Part model, mm, in its own coordinate system. A direction names the side the tool comes from. Coordinates: 2 decimals unless noted, no trailing zeros. Loops run counter-clockwise (first coordinate to the right, second up) from the corner with the lowest first, then second, coordinate; pieces in that order, holes last. Notation, with made-up numbers: (77.5, -31.5) - (112.5, -31.5) arc R29 ccw to (112.5, -3.5) - close; hole circle Ø2 at (26, 47). An arc over 180 degrees is marked (long way). Use a Markdown table: item, result. Add a question column.
1) Tool access for faces 4 (the face through (-2.5, -1.1, 8.7)), 5 (the face through (12, -7, 8)), 6 (the face through (13, 5, 8)), 7 (the face through (-1, -7, 8)), 8 (the face through (1.5, -1.1, 8.7)): list every direction of +Z, -Z, +X, -X, +Y, -Y with a clear straight run to the whole face (end or side of a thin tool).
2) Band-saw the part on C-C (x = 1). Give the cut face in (y, z), plus the area to 3 significant figures.
3) Drop flat-ended pins along their axis: P1, Ø2, axis at x = -0.5, z = 9, coming from the -Y side; P2, Ø1, axis at x = -17.5, y = -8.5, coming from the +Z side; P3, Ø2, axis at x = 11.5, z = 5.5, coming from the +Y side; P4, Ø1, axis at y = -9.5, z = 4, coming from the +X side. Give the stop position or say it passes through.
4) Band-saw the part on D-D (z = 16.25). Give the cut face in (x, y), plus the area to 3 significant figures.
5) Probe probe 1 along Y at (x, z) = (13.5, 11.85); probe 2 along X at (y, z) = (4, 9); probe 3 along Z at (x, y) = (3, 9). List the from-to ranges inside material, lowest first. Write a range as [from, to].
6) Pull direction X, two halves, no side cores. Call faces 1 (the face through (-5, -2, 0)), 2 (the face through (10.5, -0.9, 8.7)), 3 (the face through (-24.5, -9, 1)): +X half, -X half, draft (parallel to the pull), parting line (faces both ways), or undercut.
7) Band-saw the part on B-B (z = 5.25). Give the cut face in (x, y), plus the area to 4 significant figures.
8) Band-saw the part on A-A (z = 11.85). Give the cut face in (x, y).
from build123d import *

# Parameters (mm, degrees)
ESBO_O1_W                  = 10
ESBO_O1_H                  = 4
RESSALTO_EXTRUS_O1_DEPTH   = 3
ESBO_O1_8_W                = 4
ESBO_O1_8_H                = 12
RESSALTO_EXTRUS_O2_DEPTH   = 18
CORTE_EXTRUS_O1_DEPTH      = 47.968074263
CORTE_EXTRUS_O1_DEPTH_BACK = 47.968074263
ESBO_O2_R                  = 3
ESBO_O1_9_W                = 10
ESBO_O1_9_H                = 4
RESSALTO_EXTRUS_O3_DEPTH   = 8
CHANFRO1_SIZE              = 5


with BuildPart() as part:
    # Esboço1 → Ressalto-extrusão1 (new body)
    # profile 1 of 2: a face of its own
    with BuildSketch(Plane.XY):
        Polygon((-24.5, -15), (-24.5, -19), (-15.5, -19), (4.5, -19), (4.5, -15), (14.5, -15), (14.5, -7), (10.5, -7), (10.5, 5), (14.5, 5), (14.5, 15), (1.5, 15), (-1.605263158, 15), (-24.5, 0), align=None)
        with BuildLine():
            ThreePointArc((-15.5, -16.5), (-16.560660172, -16.060660172), (-17, -15))
            ThreePointArc((-17, -15), (-15.5, -13.5), (-14, -15))
            ThreePointArc((-14, -15), (-14.439339828, -16.060660172), (-15.5, -16.5))
        make_face(mode=Mode.SUBTRACT)
        Polygon((-2.5, 5), (1.5, 5), (1.5, -7), (-2.5, -7), (-2.5, 0), align=None, mode=Mode.SUBTRACT)
    # profile 2 of 2: a face of its own
    with BuildSketch(Plane.XY):
        with Locations((9.5, -17)):
            Rectangle(ESBO_O1_W, ESBO_O1_H)
    extrude(amount=RESSALTO_EXTRUS_O1_DEPTH)

    # Esboço1<8> → Ressalto-extrusão2 (add)
    with BuildSketch(Plane.XY):
        Polygon((10.5, -7), (14.5, -7), (14.5, -2), (14.5, 5), (10.5, 5), align=None)
        with Locations((-0.5, -1)):
            Rectangle(ESBO_O1_8_W, ESBO_O1_8_H)
    extrude(amount=RESSALTO_EXTRUS_O2_DEPTH)

    # Esboço2 → Corte-extrusão1 (cut, two sides: drawn at the far end of the back side and taken through both)
    with BuildSketch(Plane(origin=(14.5, 0, 0), x_dir=(0, 0, -1), z_dir=(1, 0, 0)).offset(-CORTE_EXTRUS_O1_DEPTH_BACK)):
        with BuildLine():
            ThreePointArc((-18, -1), (-16.652343178, 2.841874542), (-13.2, 5))
            Line((-13.2, 5), (-18, 5))
            Line((-18, 5), (-18, -1))
        make_face()
        with BuildLine():
            ThreePointArc((-13.2, -7), (-16.652343178, -4.841874542), (-18, -1))
            Line((-18, -1), (-18, -7))
            Line((-18, -7), (-13.2, -7))
        make_face()
        with Locations(Location((-11.85, -1, 0), (0, 0, 180))):
            Circle(ESBO_O2_R)
    extrude(amount=CORTE_EXTRUS_O1_DEPTH + CORTE_EXTRUS_O1_DEPTH_BACK, mode=Mode.SUBTRACT)

    # Esboço1<9> → Ressalto-extrusão3 (add)
    with BuildSketch(Plane.XY):
        with Locations((9.5, -17)):
            Rectangle(ESBO_O1_9_W, ESBO_O1_9_H)
    extrude(amount=RESSALTO_EXTRUS_O3_DEPTH)

    # Chanfro1
    # the kernel refuses this chamfer: 5 mm, written as the material it takes off along each edge
    with BuildSketch(Plane(origin=(27.35841494, -15, 8), x_dir=(0, 0.027495876610586317, -0.9996219169112968), z_dir=(-1, 0, 0))) as chanfro1_piece_1_section:
        Polygon((CHANFRO1_SIZE * 0.999621916911, CHANFRO1_SIZE * 0.0274958766106), (-CHANFRO1_SIZE * 0.0274958766106, CHANFRO1_SIZE * 0.999621916911), (0, 0), align=None)
    chanfro1_piece_1 = extrude(amount=35.71682988, mode=Mode.PRIVATE)
    chanfro1_piece_1 = split(chanfro1_piece_1, bisect_by=Plane(origin=(9.5, -16.652020772, 3), z_dir=(0, 0, 1)), keep=Keep.TOP, mode=Mode.PRIVATE)
    add(chanfro1_piece_1, mode=Mode.SUBTRACT)


solid = part.part
Answer block:
| question | item | result |
|---|---|---|
| 1 | face 4 | +Z, -X, +Y, -Y |
| 1 | face 5 | +Z, +X, -X |
| 1 | face 6 | +Z, +X, -X, +Y |
| 1 | face 7 | +Z, +X, -X, -Y |
| 1 | face 8 | +Z, +Y, -Y |
| 2 | outline | (-19, 0) - (15, 0) - (15, 3) - (5, 3) - (5, 13.2) arc R6.15 ccw to (-7, 13.2) - (-7, 3) - (-19, 3) - close; hole circle Ø6 at (-1, 11.85) |
| 2 | area | 239 mm2 |
| 3 | P1 | y = -7 |
| 3 | P2 | z = 3 |
| 3 | P3 | y = 5 |
| 3 | P4 | through |
| 4 | outline | (-2.5, -5.3) - (1.5, -5.3) - (1.5, 3.3) - (-2.5, 3.3) - close; (10.5, -5.3) - (14.5, -5.3) - (14.5, 3.3) - (10.5, 3.3) - close |
| 4 | area | 68.7 mm2 |
| 5 | probe 1 | [-7, -4], [2, 5] |
| 5 | probe 2 | [-2.5, 1.5], [10.5, 14.5] |
| 5 | probe 3 | [0, 3] |
| 6 | face 1 | draft |
| 6 | face 2 | undercut |
| 6 | face 3 | -X half |
| 7 | outline | (-2.5, -7) - (1.5, -7) - (1.5, 5) - (-2.5, 5) - close; (4.5, -19) - (14.5, -19) - (14.5, -17.25) - (4.5, -17.25) - close; (10.5, -7) - (14.5, -7) - (14.5, 5) - (10.5, 5) - close |
| 7 | area | 113.5 mm2 |
| 8 | outline | (-2.5, -7) - (1.5, -7) - (1.5, -4) - (-2.5, -4) - close; (-2.5, 2) - (1.5, 2) - (1.5, 5) - (-2.5, 5) - close; (10.5, -7) - (14.5, -7) - (14.5, -4) - (10.5, -4) - close; (10.5, 2) - (14.5, 2) - (14.5, 5) - (10.5, 5) - close |
